Verification items for the finished model (mm, model axes). A direction names the side the tool comes from. Coordinates: 2 decimals unless noted, no trailing zeros. Write each loop counter-clockwise with the first axis right and the second up, starting at its lowest first coordinate (ties: lowest second). Pieces come first, ordered by that corner, then holes. Notation, with made-up numbers: (16, -9) -> (35, -9) arc R6 ccw to (35, 2) -> close; hole circle Ø10 at (-9, 9). An arc over 180 degrees is marked (long way). Answer in a Markdown table with one row per item.
```python
from build123d import *

# Parameters (mm, degrees)
SKETCH6_R                 = 29
SKETCH6_R_2               = 20
INNER_RING_DEPTH          = 15
MOTOR_CONNECTOR_CUT_DEPTH = 15
SKETCH10_R                = 3.15
CUT_EXTRUDE2_DEPTH        = 55
CUT_EXTRUDE2_DEPTH_BACK   = 70
CUT_EXTRUDE4_DEPTH        = 22
CUT_EXTRUDE6_DEPTH        = 7.9
CUT_EXTRUDE5_DEPTH        = 22
SKETCH15_R                = 2.35
SKETCH15_R_2              = 1.65
BOSS_EXTRUDE1_DEPTH       = 2.9
BOSS_EXTRUDE3_DEPTH       = 2.9
CUT_EXTRUDE8_DEPTH        = 9.9
CUT_EXTRUDE7_DEPTH        = 8.9
SKETCH21_R                = 2.35
SKETCH21_R_2              = 1.65
BOSS_EXTRUDE5_DEPTH       = 2.9
SKETCH19_R                = 2.35
SKETCH19_R_2              = 1.65
BOSS_EXTRUDE4_DEPTH       = 2.9


with BuildPart() as part:
    # Sketch6 → Inner Ring (new body)
    with BuildSketch(Plane.XY):
        Circle(SKETCH6_R)
        Circle(SKETCH6_R_2, mode=Mode.SUBTRACT)
    extrude(amount=-INNER_RING_DEPTH)

    # Sketch7 → Motor Connector Cut (add)
    with BuildSketch(Plane.XY):
        with BuildLine():
            ThreePointArc((20, 0), (19.840593925, 2.52008585), (19.364916731, 5))
            Line((19.364916731, 5), (9.999996731, 5))
            Line((9.999996731, 5), (9.999996731, -5))
            Line((9.999996731, -5), (19.364916731, -5))
            ThreePointArc((19.364916731, -5), (19.840593925, -2.52008585), (20, 0))
        make_face()
        with BuildLine():
            ThreePointArc((5, 19.364916731), (0, 20), (-5, 19.364916731))
            Line((-5, 19.364916731), (-5, 9.999996731))
            Line((-5, 9.999996731), (5, 9.999996731))
            Line((5, 9.999996731), (5, 19.364916731))
        make_face()
        with BuildLine():
            Line((-9.999996731, -5), (-9.999996731, 5))
            Line((-9.999996731, 5), (-19.364916731, 5))
            ThreePointArc((-19.364916731, 5), (-20, 0), (-19.364916731, -5))
            Line((-19.364916731, -5), (-9.999996731, -5))
        make_face()
        with BuildLine():
            Line((-5, -9.999996731), (-5, -19.364916731))
            ThreePointArc((-5, -19.364916731), (0, -20), (5, -19.364916731))
            Line((5, -19.364916731), (5, -9.999996731))
            Line((5, -9.999996731), (-5, -9.999996731))
        make_face()
    extrude(amount=-MOTOR_CONNECTOR_CUT_DEPTH)

    # Sketch10 → Cut-Extrude2 (cut, two sides)
    with BuildSketch(Plane(origin=(0, 0, -15), x_dir=(-1, 0, 0), z_dir=(0, 0, -1))) as cut_extrude2_sk:
        with Locations((-17.75, 0)):
            Circle(SKETCH10_R)
        with Locations((0, 17.75)):
            Circle(SKETCH10_R)
        with Locations((17.75, 0)):
            Circle(SKETCH10_R)
        with Locations((0, -17.75)):
            Circle(SKETCH10_R)
    extrude(amount=CUT_EXTRUDE2_DEPTH, mode=Mode.SUBTRACT)
    extrude(cut_extrude2_sk.sketch, amount=-CUT_EXTRUDE2_DEPTH_BACK, mode=Mode.SUBTRACT)

    # Sketch9 → Cut-Extrude4 (cut)
    with BuildSketch(Plane(origin=(0, 0, -15), x_dir=(-1, 0, 0), z_dir=(0, 0, -1))):
        with BuildLine():
            Line((-26.38954799, 12.024631259), (-12.024631259, 26.38954799))
            ThreePointArc((-12.024631259, 26.38954799), (-20.506096654, 20.506096654), (-26.38954799, 12.024631259))
        make_face()
        with BuildLine():
            ThreePointArc((26.38954799, 12.024631259), (20.506096654, 20.506096654), (12.024631259, 26.38954799))
            Line((12.024631259, 26.38954799), (26.38954799, 12.024631259))
        make_face()
        with BuildLine():
            Line((-12.024631259, -26.38954799), (-26.38954799, -12.024631259))
            ThreePointArc((-26.38954799, -12.024631259), (-20.506096654, -20.506096654), (-12.024631259, -26.38954799))
        make_face()
        with BuildLine():
            Line((26.38954799, -12.024631259), (12.024631259, -26.38954799))
            ThreePointArc((12.024631259, -26.38954799), (20.506096654, -20.506096654), (26.38954799, -12.024631259))
        make_face()
    extrude(amount=-CUT_EXTRUDE4_DEPTH, mode=Mode.SUBTRACT)

    # Sketch16 → Cut-Extrude6 (cut)
    with BuildSketch(Plane(origin=(-19.207089624, 19.207089624, 0), x_dir=(0, 0, 1), z_dir=(-0.707106781, 0.707106781, 0))):
        with BuildLine():
            ThreePointArc((-5.15, 0), (-5.838299064, 1.661700936), (-7.5, 2.35))
            Line((-7.5, 2.35), (-7.5, -2.35))
            ThreePointArc((-7.5, -2.35), (-5.838299064, -1.661700936), (-5.15, 0))
        make_face()
        with BuildLine():
            Line((-7.5, -2.35), (-7.5, 2.35))
            ThreePointArc((-7.5, 2.35), (-9.85, 0), (-7.5, -2.35))
        make_face()
    extrude(amount=-CUT_EXTRUDE6_DEPTH, mode=Mode.SUBTRACT)

    # Sketch14 → Cut-Extrude5 (cut)
    with BuildSketch(Plane(origin=(19.207089624, 19.207089624, 0), x_dir=(0, 0, -1), z_dir=(0.707106781, 0.707106781, 0))):
        with BuildLine():
            ThreePointArc((9.85, 0), (9.161700936, 1.661700936), (7.5, 2.35))
            Line((7.5, 2.35), (7.5, -2.35))
            ThreePointArc((7.5, -2.35), (9.161700936, -1.661700936), (9.85, 0))
        make_face()
        with BuildLine():
            Line((7.5, -2.35), (7.5, 2.35))
            ThreePointArc((7.5, 2.35), (5.15, 0), (7.5, -2.35))
        make_face()
    extrude(amount=-CUT_EXTRUDE5_DEPTH, mode=Mode.SUBTRACT)

    # Sketch15 → Boss-Extrude1 (add)
    with BuildSketch(Plane(origin=(19.207089624, 19.207089624, 0), x_dir=(0, 0, -1), z_dir=(0.707106781, 0.707106781, 0))):
        with Locations((7.5, 0)):
            Circle(SKETCH15_R)
        with Locations((7.5, 0)):
            Circle(SKETCH15_R_2, mode=Mode.SUBTRACT)
    extrude(amount=-BOSS_EXTRUDE1_DEPTH)

    # Sketch17 → Boss-Extrude3 (add)
    with BuildSketch(Plane(origin=(-19.207089624, 19.207089624, 0), x_dir=(0, 0, 1), z_dir=(-0.707106781, 0.707106781, 0))):
        with BuildLine():
            ThreePointArc((-5.15, 0), (-5.838299064, 1.661700936), (-7.5, 2.35))
            Line((-7.5, 2.35), (-7.5, 1.65))
            ThreePointArc((-7.5, 1.65), (-6.333273811, 1.166726189), (-5.85, 0))
            ThreePointArc((-5.85, 0), (-6.333273811, -1.166726189), (-7.5, -1.65))
            Line((-7.5, -1.65), (-7.5, -2.35))
            ThreePointArc((-7.5, -2.35), (-5.838299064, -1.661700936), (-5.15, 0))
        make_face()
        with BuildLine():
            Line((-7.5, 1.65), (-7.5, 2.35))
            ThreePointArc((-7.5, 2.35), (-9.85, 0), (-7.5, -2.35))
            Line((-7.5, -2.35), (-7.5, -1.65))
            ThreePointArc((-7.5, -1.65), (-9.15, 0), (-7.5, 1.65))
        make_face()
    extrude(amount=-BOSS_EXTRUDE3_DEPTH)

    # Sketch20 → Cut-Extrude8 (cut)
    with BuildSketch(Plane(origin=(-19.207089624, -19.207089624, 0), x_dir=(0, 0, 1), z_dir=(-0.707106781, -0.707106781, 0))):
        with BuildLine():
            ThreePointArc((-5.15, 0), (-5.838299064, 1.661700936), (-7.5, 2.35))
            Line((-7.5, 2.35), (-7.5, -2.35))
            ThreePointArc((-7.5, -2.35), (-5.838299064, -1.661700936), (-5.15, 0))
        make_face()
        with BuildLine():
            Line((-7.5, -2.35), (-7.5, 2.35))
            ThreePointArc((-7.5, 2.35), (-9.85, 0), (-7.5, -2.35))
        make_face()
    extrude(amount=-CUT_EXTRUDE8_DEPTH, mode=Mode.SUBTRACT)

    # Sketch18 → Cut-Extrude7 (cut)
    with BuildSketch(Plane(origin=(19.207089624, -19.207089624, 0), x_dir=(0, 0, -1), z_dir=(0.707106781, -0.707106781, 0))):
        with BuildLine():
            ThreePointArc((9.85, 0), (9.161700936, 1.661700936), (7.5, 2.35))
            Line((7.5, 2.35), (7.5, -2.35))
            ThreePointArc((7.5, -2.35), (9.161700936, -1.661700936), (9.85, 0))
        make_face()
        with BuildLine():
            Line((7.5, -2.35), (7.5, 2.35))
            ThreePointArc((7.5, 2.35), (5.15, 0), (7.5, -2.35))
        make_face()
    extrude(amount=-CUT_EXTRUDE7_DEPTH, mode=Mode.SUBTRACT)

    # Sketch21 → Boss-Extrude5 (add)
    with BuildSketch(Plane(origin=(-19.207089624, -19.207089624, 0), x_dir=(0, 0, 1), z_dir=(-0.707106781, -0.707106781, 0))):
        with Locations((-7.5, 0)):
            Circle(SKETCH21_R)
        with Locations((-7.5, 0)):
            Circle(SKETCH21_R_2, mode=Mode.SUBTRACT)
    extrude(amount=-BOSS_EXTRUDE5_DEPTH)

    # Sketch19 → Boss-Extrude4 (add)
    with BuildSketch(Plane(origin=(19.207089624, -19.207089624, 0), x_dir=(0, 0, -1), z_dir=(0.707106781, -0.707106781, 0))):
        with Locations((7.5, 0)):
            Circle(SKETCH19_R)
        with Locations((7.5, 0)):
            Circle(SKETCH19_R_2, mode=Mode.SUBTRACT)
    extrude(amount=-BOSS_EXTRUDE4_DEPTH)


solid = part.part
```
1. Sectioned sample at C-C, the plane z = -3. Record the cut outline in (x, y).
Findings below:
| item | result |
|---|---|
| outline | (-26.39, -12.02) -> (-12.02, -26.39) arc R29 ccw to (12.02, -26.39) -> (26.39, -12.02) arc R29 ccw to (26.39, 12.02) -> (12.02, 26.39) arc R29 ccw to (-12.02, 26.39) -> (-26.39, 12.02) arc R29 ccw to start; hole circle Ø6.3 at (-17.75, 0); hole (-19.36, -5) arc R20 ccw to (-5, -19.36) -> (-5, -10) -> (5, -10) -> (5, -19.36) arc R20 ccw to (19.36, -5) -> (10, -5) -> (10, 5) -> (19.36, 5) arc R20 ccw to (5, 19.36) -> (5, 10) -> (-5, 10) -> (-5, 19.36) arc R20 ccw to (-19.36, 5) -> (-10, 5) -> (-10, -5) -> close; hole circle Ø6.3 at (0, -17.75); hole circle Ø6.3 at (0, 17.75); hole circle Ø6.3 at (17.75, 0) |
2. Material ranges on probe 1 along Y at (x, z) = (0, -10.25); probe 2 along Y at (x, z) = (-11, -12.5); probe 3 along X at (y, z) = (18, -1.5), recorded low to high. Write a range as from..to.
Findings below:
| item | result |
|---|---|
| probe 1 | y = -29..-20.9, -14.6..-10, 10..14.6, 20.9..29 |
| probe 2 | y = -26.83..-16.7, -5..5, 16.7..26.83 |
| probe 3 | x = -20.41..-8.72, -5..-3.14, 3.14..5, 8.72..20.41 |
3. Sectioned sample at A-A, the plane x = 0. Record the cut outline in (y, z), and give its area (3 significant figures).
Findings below:
| item | result |
|---|---|
| outline | (-29, -15) -> (-20.9, -15) -> (-20.9, 0) -> (-29, 0) -> close; (-14.6, -15) -> (-10, -15) -> (-10, 0) -> (-14.6, 0) -> close; (10, -15) -> (14.6, -15) -> (14.6, 0) -> (10, 0) -> close; (20.9, -15) -> (29, -15) -> (29, 0) -> (20.9, 0) -> close |
| area | 381 mm² |
4. Go/stop test with flat-tipped pins: pin 1 (6 mm diameter, centred on y = 0.5, z = -9, fed in from +X); pin 2 (4.5 mm diameter, centred on y = -15.5, z = -4.5, fed in from -X); pin 3 (8 mm diameter, centred on x = 2, z = -4.5, fed in from -Y). Record where each tip stops, or that it passes through.
Findings below:
| item | result |
|---|---|
| pin 1 | stops at x = 29 |
| pin 2 | stops at x = -25.16 |
| pin 3 | stops at y = -29 |
5. Release check for a two-part mould opening along Y. For faces 4 (the face through (20.703, 17.712, -7.395)), 5 (the face through (-29, 0, -7)), 6 (the face through (0, -29, -7)), 7 (the face through (19, -17.4, -6.3)) record: released by +Y, released by -Y, zero draft, split by the parting line, or undercut.
Findings below:
| item | result |
|---|---|
| face 4 | released by +Y |
| face 5 | split by the parting line |
| face 6 | released by -Y |
| face 7 | undercut |
6. Access from +Z, -Z, +X, -X, +Y, -Y to the whole of each face (thin tool, end or side, straight path). Record for faces 1 (the face through (-18.241, 16.072, -6.488)), 2 (the face through (-10, 0, -7)), 3 (the face through (17.712, -20.703, -7.395)).
Findings below:
| item | result |
|---|---|
| face 1 | none |
| face 2 | +Z, -Z |
| face 3 | +Z, -Z, +X, -Y |
7. Sectioned sample at D-D, the plane y = -7.5. Record the cut outline in (x, z), and give its area (3 significant figures).
Findings below:
| item | result |
|---|---|
| outline | (-28.01, -15) -> (-18.54, -15) -> (-18.54, 0) -> (-28.01, 0) -> close; (18.54, -15) -> (28.01, -15) -> (28.01, 0) -> (18.54, 0) -> close |
| area | 284 mm² |
